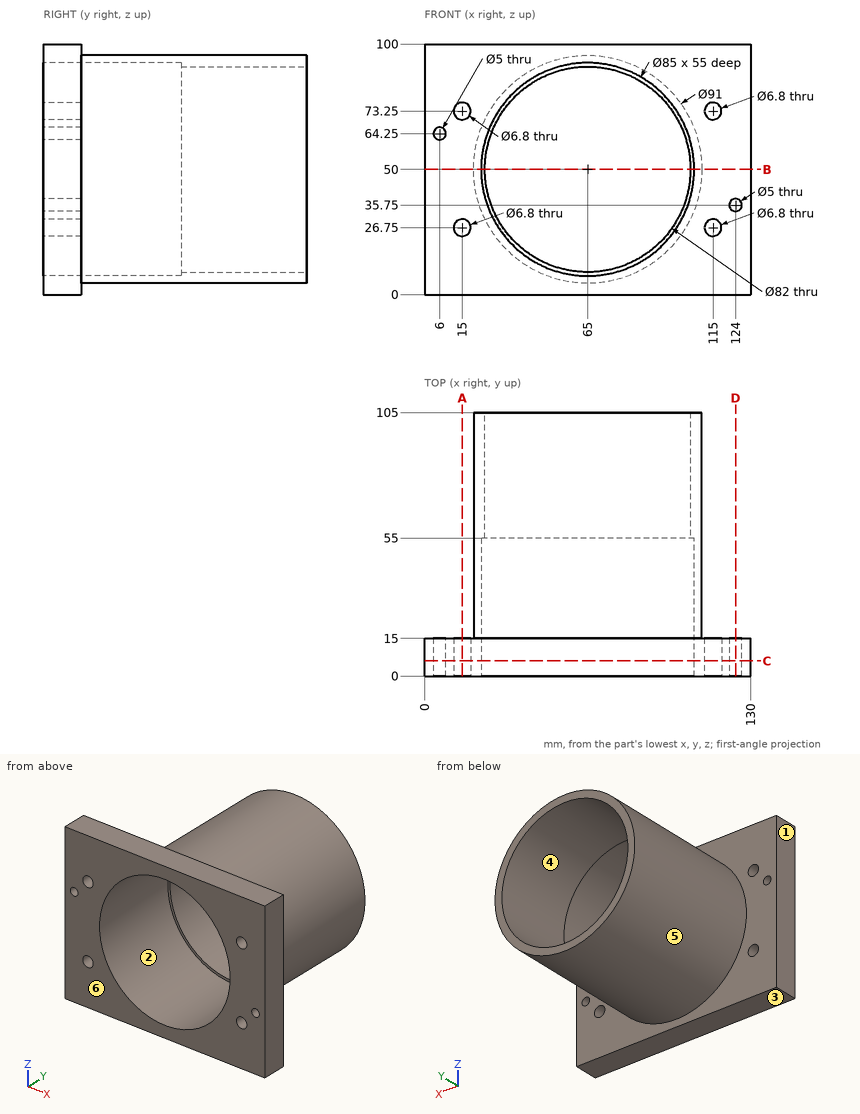
Job drawing, mm, ordinate dimensions from the low corner. One solid piece. A direction names the side the tool comes from. Coordinates: 2 decimals unless noted, no trailing zeros. Order: outer loops, then holes, each group sorted by start corner. A loop starts at its lowest first (then second) coordinate and runs counter-clockwise, first axis right, second up. Notation, with made-up numbers: M 47.5,67.5 L 74.5,67.5 A29 cw 74.5,101.5 Z; hole C -7.5,24 d9. An arc over 180 degrees is marked long. Return JSON: item names as keys, results as strings.
1. Saw through at A-A (x = 15). Give the cut face in (y, z), and give its area (3 significant figures).
Ans:
{"outline": "M 0,0 L 15,0 L 15,23.35 L 0,23.35 Z; M 0,30.15 L 15,30.15 L 15,69.85 L 0,69.85 Z; M 0,76.65 L 15,76.65 L 15,100 L 0,100 Z", "area": "1,300 mm^2"}
2. Tool access for the marked faces 5 and 6: list every direction of +Z, -Z, +X, -X, +Y, -Y with a clear straight run to the whole face (end or side of a thin tool).
Ans:
{"face 5": "+Y", "face 6": "+Z, -Z, +X, -X, -Y"}
3. Pull direction Z, two halves, no side cores. Call the marked faces 1, 2, 3 and 4: +Z half, -Z half, draft (parallel to the pull), parting line (faces both ways), or undercut.
Ans:
{"face 1": "draft", "face 2": "undercut", "face 3": "-Z half", "face 4": "undercut"}
4. Saw through at D-D (x = 124). Give the cut face in (y, z), and give its area (4 significant figures).
Ans:
{"outline": "M 0,0 L 15,0 L 15,33.25 L 0,33.25 Z; M 0,38.25 L 15,38.25 L 15,100 L 0,100 Z", "area": "1,425 mm^2"}
5. Saw through at C-C (y = 6). Give the cut face in (x, z).
Ans:
{"outline": "M 0,0 L 130,0 L 130,100 L 0,100 Z; hole C 6,64.25 d5; hole C 15,26.75 d6.8; hole C 15,73.25 d6.8; hole C 65,50 d85; hole C 115,26.75 d6.8; hole C 115,73.25 d6.8; hole C 124,35.75 d5"}
6. Flat gauge pins, fed straight in: pin 1 (11 mm diameter, centred on x = 115, z = 26.75, fed in from -Y); pin 2 (3 mm diameter, centred on y = 77, z = 51.5, fed in from +X); pin 3 (5 mm diameter, centred on x = 48, y = 62.5, fed in from -Z); pin 4 (5 mm diameter, centred on y = 19.5, z = 86, fed in from -X). Where does each tip first touch, or does it go through?
Ans:
{"pin 1": "y = 0", "pin 2": "x = 110.5", "pin 3": "z = 6.87", "pin 4": "x = 34.21"}
7. Drill centre lines: probe 1 along Z at (x, y) = (15, 3.5); probe 2 along X at (y, z) = (92, 50); probe 3 along Z at (x, y) = (6, 5). Where is each one in solid material? Low to high.
Ans:
{"probe 1": "0 to 23.35, 30.15 to 69.85, 76.65 to 100", "probe 2": "19.5 to 24, 106 to 110.5", "probe 3": "0 to 61.75, 66.75 to 100"}
8. Saw through at B-B (z = 50). Give the cut face in (x, y).
Ans:
{"outline": "M 0,0 L 22.5,0 L 22.5,55 L 24,55 L 24,105 L 19.5,105 L 19.5,15 L 0,15 Z; M 106,55 L 107.5,55 L 107.5,0 L 130,0 L 130,15 L 110.5,15 L 110.5,105 L 106,105 Z"}
